Check sheet for the modelled part. Datum: model origin and axes. Units: mm. A direction names the side the tool comes from. Coordinates: 2 decimals unless noted, no trailing zeros. Loops run counter-clockwise (first coordinate to the right, second up) from the corner with the lowest first, then second, coordinate; pieces in that order, holes last. Notation, with made-up numbers: (29.5, 49) - (76.5, 49) arc R35 ccw to (76.5, 84) - close; hole circle Ø5 at (16.25, -30.75). An arc over 180 degrees is marked (long way). Write each question's results on one line, items separated by ' | '. Start each with the question number.
1. Draft check along X on faces 1 (the face through (3.89, 8.96, 7.48)), 2 (the face through (0, 6, 6)), 3 (the face through (40, 6, 6)), 4 (the face through (21.75, 10, 18)). Enter one of: released by +X, released by -X, zero draft, split by the parting line, or undercut.
2. Cross-section at D-D (y = 7). Record the cut outline in (x, z), and give its area (3 significant figures).
3. Tool access check on faces 5 (the face through (3.35, 2.27, 3.23)), 6 (the face through (19.9, 7.6, 15)), 7 (the face through (20, 8, 17)), 8 (the face through (5, 6, 15)). Record the directions out of +Z, -Z, +X, -X, +Y, -Y that give a thin tool (end or side, any length) a straight path to the whole face; none if there is none.
4. Cross-section at C-C (z = 18.75). Record the cut outline in (x, y), and give its area (3 significant figures).
5. Thickness scan on line 1 (X direction, y = 7, z = 6); line 2 (X direction, y = 1.6, z = 6); line 3 (X direction, y = 10.25, z = 2.5). Record the ranges inside material, lowest first. Write a range as [from, to].
6. Gauge pin test, flat ends, axial feed: P1, Ø1, axis at x = 19.5, z = 18, coming from the +Y side; P2, Ø1.5, axis at x = 34, y = 9.5, coming from the +Z side; P3, Ø2.5, axis at x = 35.67, z = 6, coming from the -Y side; P4, Ø10.5, axis at x = 20.5, z = 5, coming from the +Y side. Record the tip position at first contact, or that the pin passes through.
7. Cross-section at B-B (x = 23.25). Record the cut outline in (y, z).
8. Cross-section at A-A (y = 9.5). Record the cut outline in (x, z), and give its area (3 significant figures).
```python
from build123d import *

# Parameters (mm, degrees)
SKETCH_1_W          = 40
SKETCH_1_H          = 20
SKETCH_1_R          = 1.6
EXTRUDE_1_DEPTH     = 12
SKETCH_2_W          = 13
SKETCH_2_H          = 15
CUT_EXTRUDE_1_DEPTH = 6.2
SKETCH_3_W          = 3.5
SKETCH_3_H          = 5
CUT_EXTRUDE_2_DEPTH = 4
CHAMFER_1_SIZE      = 10
FILLET_1_R          = 2
SKETCH_4_R          = 0.7
CUT_EXTRUDE_3_DEPTH = 46.149086369
SKETCH_5_R          = 3
CUT_EXTRUDE_4_DEPTH = 4
CHAMFER_2_SIZE      = 2


with BuildPart() as part:
    # 草图1 → 凸台-拉伸1 (new body)
    with BuildSketch(Plane(origin=(0, 0, 0), x_dir=(1, 0, 0), z_dir=(0, 1, 0))):
        with Locations((20, -10)):
            Rectangle(SKETCH_1_W, SKETCH_1_H)
        with Locations(Location((4.5, -6, 0), (0, 0, 270))):
            Circle(SKETCH_1_R, mode=Mode.SUBTRACT)
        with Locations(Location((35.672897196, -6, 0), (0, 0, 270))):
            Circle(SKETCH_1_R, mode=Mode.SUBTRACT)
    extrude(amount=EXTRUDE_1_DEPTH)

    # 草图2 → 切除-拉伸1 (cut)
    with BuildSketch(Plane(origin=(0, 12, 0), x_dir=(1, 0, 0), z_dir=(0, 1, 0))):
        with Locations((20, -7.5)):
            Rectangle(SKETCH_2_W, SKETCH_2_H)
    extrude(amount=-CUT_EXTRUDE_1_DEPTH, mode=Mode.SUBTRACT)

    # 草图3 → 切除-拉伸2 (cut)
    with BuildSketch(Plane(origin=(0, 12, 0), x_dir=(1, 0, 0), z_dir=(0, 1, 0))):
        with Locations((20, -17.5)):
            Rectangle(SKETCH_3_W, SKETCH_3_H)
    extrude(amount=-CUT_EXTRUDE_2_DEPTH, mode=Mode.SUBTRACT)

    # 倒角1
    chamfer_1_edges = [part.edges().sort_by_distance(p)[0] for p in [
        (40, 6, 20),
        (0, 6, 20),
    ]]
    chamfer(chamfer_1_edges, length=CHAMFER_1_SIZE)

    # 圆角1
    fillet_1_edges = [part.edges().sort_by_distance(p)[0] for p in [
        (40, 6, 10),
        (10, 6, 20),
        (30, 6, 20),
        (0, 6, 10),
        (0, 6, 0),
        (40, 6, 0),
    ]]
    fillet(fillet_1_edges, radius=FILLET_1_R)

    # 草图4 → 切除-拉伸3 (cut, through all)
    with BuildSketch(Plane(origin=(0, 5.8, 0), x_dir=(1, 0, 0), z_dir=(0, 1, 0))):
        with Locations(Location((16.75, -5, 0), (0, 0, 270))):
            Circle(SKETCH_4_R)
        with Locations(Location((23.25, -5, 0), (0, 0, 270))):
            Circle(SKETCH_4_R)
    extrude(amount=-CUT_EXTRUDE_3_DEPTH, mode=Mode.SUBTRACT)

    # 草图5 → 切除-拉伸4 (cut)
    with BuildSketch(Plane(origin=(0, 0, 0), x_dir=(-1, 0, 0), z_dir=(0, -1, 0))):
        with Locations(Location((-35.672897196, -6, 0), (0, 0, 90))):
            Circle(SKETCH_5_R)
        with Locations(Location((-4.5, -6, 0), (0, 0, 90))):
            Circle(SKETCH_5_R)
    extrude(amount=-CUT_EXTRUDE_4_DEPTH, mode=Mode.SUBTRACT)

    # 倒角2
    # the kernel refuses this chamfer: 2 mm, written as the material it takes off along each edge
    with BuildSketch(Plane(origin=(35.672897196, 4, 6), x_dir=(0, 0, 1), z_dir=(1, 0, 0))) as chamfer_2_piece_1_section:
        Polygon((1.6 + CHAMFER_2_SIZE, 0), (1.6, -CHAMFER_2_SIZE), (1.6, 0), align=None)
    chamfer_2_piece_1 = revolve(axis=Axis((35.672897196, 4, 6), (0, -1, 0)), mode=Mode.PRIVATE)
    chamfer_2_piece_1 = chamfer_2_piece_1 & Plane(origin=(35.672897196, 5.307163584, 6), x_dir=(0, 0, -1), z_dir=(0, -1, 0)) * Cylinder(3, 15, mode=Mode.PRIVATE)
    add(chamfer_2_piece_1, mode=Mode.SUBTRACT)
    with BuildSketch(Plane(origin=(4.5, 4, 6), x_dir=(0, 0, 1), z_dir=(1, 0, 0))) as chamfer_2_piece_2_section:
        Polygon((1.6 + CHAMFER_2_SIZE, 0), (1.6, -CHAMFER_2_SIZE), (1.6, 0), align=None)
    chamfer_2_piece_2 = revolve(axis=Axis((4.5, 4, 6), (0, -1, 0)), mode=Mode.PRIVATE)
    chamfer_2_piece_2 = chamfer_2_piece_2 & Plane(origin=(4.5, 5.307163584, 6), x_dir=(0, 0, -1), z_dir=(0, -1, 0)) * Cylinder(3, 15, mode=Mode.PRIVATE)
    add(chamfer_2_piece_2, mode=Mode.SUBTRACT)


solid = part.part
```
Established:
1) face 1: undercut | face 2: released by -X | face 3: released by +X | face 4: undercut
2) outline: (0, 2) arc R2 ccw to (2, 0) - (13.5, 0) - (13.5, 15) - (26.5, 15) - (26.5, 0) - (38, 0) arc R2 ccw to (40, 2) - (40, 9.17) arc R2 ccw to (39.41, 10.59) - (30.59, 19.41) arc R2 ccw to (29.17, 20) - (10.83, 20) arc R2 ccw to (9.41, 19.41) - (0.59, 10.59) arc R2 ccw to (0, 9.17) - close; hole circle Ø3.2 at (4.5, 6); hole circle Ø3.2 at (35.67, 6) | area: 487 mm^2
3) face 5: -Y | face 6: -Z, +Y | face 7: +Z, -Z, +Y | face 8: +Z, -X, +Y, -Y
4) outline: (8.75, 0) - (31.25, 0) - (31.25, 12) - (21.75, 12) - (21.75, 8) - (18.25, 8) - (18.25, 12) - (8.75, 12) - close | area: 256 mm^2
5) line 1: [0, 2.9], [6.1, 13.5], [26.5, 34.07], [37.27, 40] | line 2: [0, 1.5], [7.5, 32.67], [38.67, 40] | line 3: [0, 13.5], [26.5, 40]
6) P1: y = 8 | P2: z = 16.75 | P3: through | P4: y = 5.8
7) outline: (0, 0) - (5.8, 0) - (5.8, 4.3) - (0, 4.3) - close; (0, 5.7) - (5.8, 5.7) - (5.8, 15) - (12, 15) - (12, 20) - (0, 20) - close
8) outline: (0, 2) arc R2 ccw to (2, 0) - (13.5, 0) - (13.5, 15) - (18.25, 15) - (18.25, 20) - (10.83, 20) arc R2 ccw to (9.41, 19.41) - (0.59, 10.59) arc R2 ccw to (0, 9.17) - close; (21.75, 15) - (26.5, 15) - (26.5, 0) - (38, 0) arc R2 ccw to (40, 2) - (40, 9.17) arc R2 ccw to (39.41, 10.59) - (30.59, 19.41) arc R2 ccw to (29.17, 20) - (21.75, 20) - close; hole circle Ø3.2 at (4.5, 6); hole circle Ø3.2 at (35.67, 6) | area: 469 mm^2
